Autodesk Inventor part; units mm, degrees
ref_plane "Work Plane2" through (3.35, 0, 0) normal (0, 0, -1) x (1, 0, 0)
ref_plane "YZ Plane" through (0, 0, 0) normal (1, 0, 0) x (0, 1, 0)
ref_plane "XZ Plane" through (0, 0, 0) normal (0, 1, 0) x (-1, 0, 0)
sketch "Эскиз1" plane through (0, 0, 0) normal (0, 0, 1) x (1, 0, 0)
  line L0 (1.4, 0) -> (30, 0)
  line L1 (11, 1.5) -> (10.6933, 1.5)
  line L2 (0, 2.8) -> (0, 1.4)
  line L3 (0, 1.4) -> (0.8921, 0.9552)
  line L4 (0.8921, 0.9552) -> (1.4, 0)
  line L5 (-6.73, 0) -> (40.38, 0)
  line L6 (0, -0.56) -> (0, 3.36)
  line L7 (0, 2.8) -> (0.35, 2.8)
  line L8 (0.35, 2.8) -> (1.65, 1.5)
  line L9 (11, 1.5) -> (1.65, 1.5) construction
  line L10 (1.65, 1.5) -> (33.65, 1.5)
  line L11 (33.65, 1.5) -> (33.65, 0)
  line L12 (33.65, 0) -> (30, 0)
  dimension "d4" = 2.8
  dimension "d5" = 26.5
  dimension "d6" = 62
  dimension "d7" = 1.4
  dimension "d8" = 0.3067
  dimension "d12" = 5.6
  dimension "d13" = 45
  dimension "d24" = 1.65
  dimension "d96" = 32
revolve "Базовый элемент" add sketch "Эскиз1" angle 360 about axis through (1.4, 0, 0) along (1, 0, 0) contours L4 L3 L2 L7 L8 L10 L1 L11 L5 L0
sketch "Эскиз2" plane through (0, 0, 0) normal (-1, 0, 0) x (0, 0, 1)
  line L0 (0, 1.4) -> (0, 0) construction
  line L1 (0, 0) -> (1.4, 0) construction
  arc A0 (0.42, 0) -> (0, 0.42) centre (0, 0) ccw construction
  arc A1 (0.49, 0) -> (0, 0.49) centre (0, 0) ccw construction
  arc A2 (1.3838, 0.2125) -> (0.2125, 1.3838) centre (0, 0) ccw
  line L2 (0, 0) -> (0.9899, 0.9899) construction
  line L3 (0.2125, 1.3838) -> (0.241, 0.4266)
  line L4 (1.3838, 0.2125) -> (0.4266, 0.241)
  arc A3 (0.2125, 1.3838) -> (0, 1.4) centre (0, 0) ccw
  arc A4 (1.4, 0) -> (1.3838, 0.2125) centre (0, 0) ccw
  line L5 (0, -3.92) -> (0, 3.92)
  line L6 (-3.92, 0) -> (3.92, 0)
  arc A5 (0.2125, -1.3838) -> (1.3838, -0.2125) centre (0, 0) ccw
  line L7 (0.2125, -1.3838) -> (0.241, -0.4266)
  line L8 (1.3838, -0.2125) -> (0.4266, -0.241)
  arc A6 (0, -1.4) -> (0.2125, -1.3838) centre (0, 0) ccw
  arc A7 (1.3838, -0.2125) -> (1.4, 0) centre (0, 0) ccw
  arc A8 (-0.2125, 1.3838) -> (-1.3838, 0.2125) centre (0, 0) ccw
  line L9 (-0.2125, 1.3838) -> (-0.241, 0.4266)
  line L10 (-1.3838, 0.2125) -> (-0.4266, 0.241)
  arc A9 (0, 1.4) -> (-0.2125, 1.3838) centre (0, 0) ccw
  arc A10 (-1.3838, 0.2125) -> (-1.4, 0) centre (0, 0) ccw
  arc A11 (-0.2125, -1.3838) -> (0, -1.4) centre (0, 0) ccw
  arc A12 (-1.3838, -0.2125) -> (-0.2125, -1.3838) centre (0, 0) ccw
  arc A13 (-1.4, 0) -> (-1.3838, -0.2125) centre (0, 0) ccw
  line L11 (-1.3838, -0.2125) -> (-0.4266, -0.241)
  line L12 (-0.2125, -1.3838) -> (-0.241, -0.4266)
  arc A14 (0.241, 0.4266) -> (0.4266, 0.241) centre (0.4323, 0.4323) ccw
  arc A15 (0.4266, -0.241) -> (0.241, -0.4266) centre (0.4323, -0.4323) ccw
  arc A16 (-0.4266, 0.241) -> (-0.241, 0.4266) centre (-0.4323, 0.4323) ccw
  arc A17 (-0.241, -0.4266) -> (-0.4266, -0.241) centre (-0.4323, -0.4323) ccw
  point P0 (0.9899, -0.9899)
  point P1 (-0.9899, 0.9899)
  point P2 (-0.9899, -0.9899)
  dimension "d17" = 0.84
  dimension "d18" = 0.98
  dimension "d19" = 2.8
  dimension "d20" = 45
  dimension "d21" = 0.2125
extrude "Паз" add sketch "Эскиз2" against normal up to next draft 5 contours L4 A14 L3 A2 | A5 L7 A15 L8 | L9 A16 L10 A8 | A12 L11 A17 L12
fillet "Сопряжение1" radius 0.085 4 edges at (0, 1.4, 0) (0, 0, -1.4) (0, -1.4, 0) (0, 0, 1.4)
thread "Резьба"
ref_plane "Work Plane2" through (3.35, 0, 0) normal (0, 0, -1) x (1, 0, 0)
equation "\"d17\" = 0.3 * SDM"
equation "\"d18\" = 0.35 * SDM"
equation "\"d19\" = SDM"
equation "\"d21\" = 0.5 * SBR"
equation "\"d4\" = SDM"
equation "\"d7\" = INTI"
equation "\"d8\" = GAL"
equation "\"d12\" = KOD"
equation "\"d13\" = 0.5 * SEWI"
equation "\"d24\" = KOH"
equation "\"d23\" = 0.2 * SBR"
equation "\"d10\" = d96"
equation "\"GEL\" = 19"
equation "\"GAL\" = 0.61345 * PTC"
equation "\"SPD\" = NND - 1.2269 * PTC"
equation "\"KOD\" = 5.6"
equation "\"KOH\" = 1.65"
equation "\"SBR\" = 0.425"
equation "\"INTI\" = 1.4"
equation "\"SDM\" = 2.8"
equation "\"GD\" = NND"
equation "\"BDM\" = NND"
equation "\"SEWI\" = 90deg"
equation "\"d9\" = SDM"
equation "\"GUL\" = 0.61345 * PTC"
equation "\"TOA\" = 30deg"
equation "\"EPV\" = 3.15"
equation "\"THREADDIA\" = 3"
equation "\"FAWI\" = 45deg"
equation "\"RR\" = 0.1 * NND"
equation "\"PTC\" = 0.5"
equation "\"NND\" = 3"
equation "\"GD1\" = THREADDIA - 1.2269 * PTC"
properties part number "Винт 2.M3-6gx30 ГОСТ 17475-80" material "Сталь, мягкая"
Geometry check sheet. Reference: the model listing, model coordinates, mm. A direction names the side the tool comes from. Round coordinates to 2 decimals unless told otherwise and drop trailing zeros. Write each loop counter-clockwise with the first axis right and the second up, starting at its lowest first coordinate (ties: lowest second). Pieces come first, ordered by that corner, then holes. Notation, with made-up numbers: (18, 58.5) - (29, 58.5) arc R20 ccw to (29, 68.5) - close; hole circle Ø5 at (-38, 74). An arc over 180 degrees is marked (long way). One line per item, written item: value.
1. Depth check by flat-ended pin: pin 1 Ø1 at (x, y) = (4, 0.5) entering from -Z; pin 2 Ø1 at (x, z) = (5.5, -1.5) entering from -Y; pin 3 Ø3 at (x, y) = (14.5, -0.5) entering from +Z. Enter the tip coordinate at first touch or a pass-through.
The answers:
pin 1: stops at z = -1.5
pin 2: stops at y = -1.12
pin 3: stops at z = 1.5
2. Mould release check, pull along Y, two halves, no side actions. Record for faces 1 (the face through (0.2, -2.8, 0.1)), 2 (the face through (0, 1, -1)), 3 (the face through (1.312, -0.122, -0.112)): released by +Y, released by -Y, zero draft, split by the parting line, or undercut.
The answers:
face 1: split by the parting line
face 2: zero draft
face 3: undercut
3. Cross-section at A-A on x = 3.5. Record the boundary of the cut face in (y, z), and give its area (3 significant figures).
The answers:
outline: circle Ø3 at (0, 0)
area: 7.07 mm^2
4. Set-up check for faces 4 (the face through (17.87, -1.5, 0.07)), 5 (the face through (33.65, 0, 0)): record each of +Z, -Z, +X, -X, +Y, -Y from which the full face is reachable in a straight line by a thin tool's end or side.
The answers:
face 4: +X
face 5: +Z, -Z, +X, +Y, -Y
5. Scan lines: L1, parallel to Y at x = 22, z = -0.6; L2, parallel to Z at x = 25, y = -0.45; L3, parallel to Y at x = 7, z = -0.1. Record each from-to range of solid material in increasing order.
The answers:
L1: y = -1.37 to 1.37
L2: z = -1.43 to 1.43
L3: y = -1.5 to 1.5
